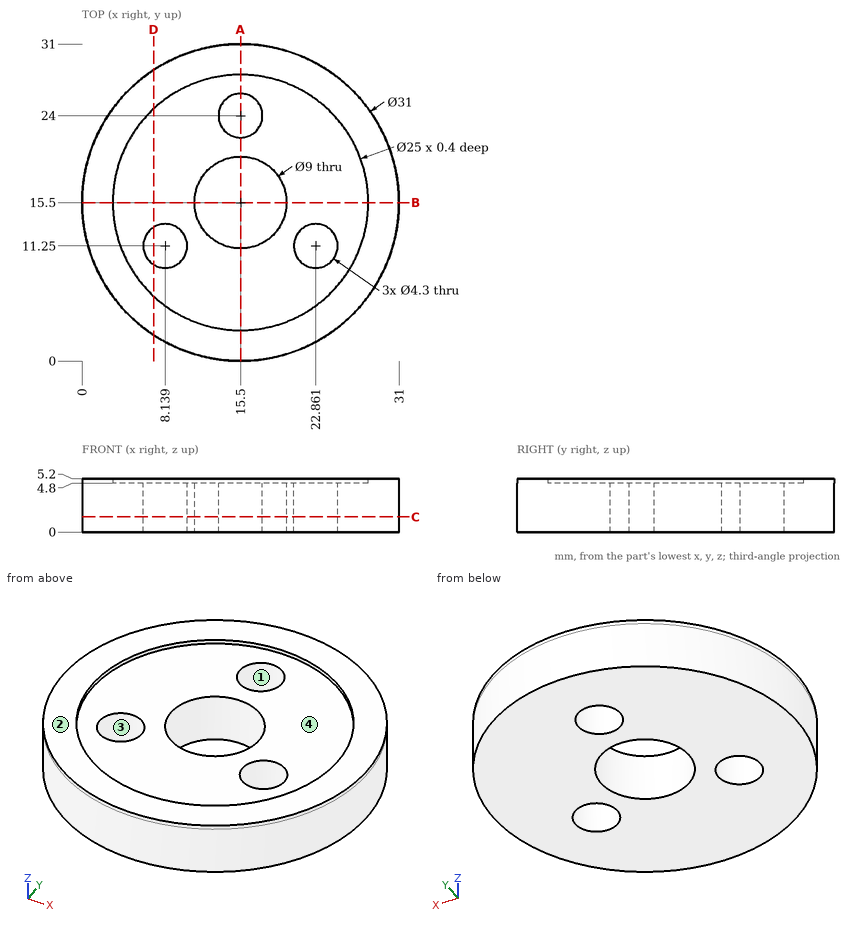
Here's the drawing with two shaded views (mm, measured from the low corner). I have some questions. A direction names the side the tool comes from. Give positions to 0.01 mm unless a question says otherwise; leave off trailing zeros. Order: outer loops, then holes, each group sorted by start corner. A loop starts at its lowest first (then second) coordinate and runs counter-clockwise, first axis right, second up. Notation, with made-up numbers: M -25,5.5 L 1,5.5 A36 ccw 1,41.5 Z; hole C -34,36 d5. An arc over 180 degrees is marked long. Answer as a JSON object with one key per item and string values. Group by question number.
1) On a 3-axis mill with a long thin cutter (end or side, diameter ignored), from which of +Z, -Z, +X, -X, +Y, -Y can I reach the whole of each face in a straight line? I mean the marked faces 3 and 4. Say none if no direction works.
2) Suppose I cut it at B-B, the plane y = 15.5. Write out the boundary of the cut face in (x, z), plus the area to 3 significant figures.
3) Suppose I cut it at D-D, the plane x = 7. Write out the boundary of the cut face in (y, z) (1 decimal), plus the area to 3 significant figures.
4) Suppose I cut it at C-C, the plane z = 1.5. Write out the boundary of the cut face in (x, y), plus the area to 3 significant figures.
5) Please list where these lines run through material, in increasing order: L1, parallel to Y at x = 15.5, z = 3.35; L2, parallel to Z at x = 25, y = 8.5; L3, parallel to X at y = 17, z = 4.5. Write a range as [from, to].
6) I'm going to push flat-ended pins straight in: pin 1 Ø2 at (x, y) = (23, 13) entering from +Z; pin 2 Ø1.5 at (x, z) = (14.5, 3.5) entering from -Y; pin 3 Ø3 at (x, z) = (8, 1.5) entering from -Y. Where does each tip first touch, or does it pass through?
7) We'd pull the mould along Y, two halves only. Please class the marked faces 1 and 2: pulls with the +Y half, pulls with the -Y half, needs draft (parallel to the pull), parting line crosses it, or undercut.
8) Suppose I cut it at A-A, the plane x = 15.5. Write out the boundary of the cut face in (y, z).
Results found:
{
 "1": {"face 3": "+Z, -Z", "face 4": "+Z"},
 "2": {"outline": "M 0,0 L 11,0 L 11,4.8 L 3,4.8 L 3,5.2 L 0,5.2 Z; M 20,0 L 31,0 L 31,5.2 L 28,5.2 L 28,4.8 L 20,4.8 Z", "area": "108 mm²"},
 "3": {"outline": "M 2.5,0 L 9.4,0 L 9.4,4.8 L 6.3,4.8 L 6.3,5.2 L 2.5,5.2 Z; M 13.1,0 L 28.5,0 L 28.5,5.2 L 24.7,5.2 L 24.7,4.8 L 13.1,4.8 Z", "area": "110 mm²"},
 "4": {"outline": "C 15.5,15.5 d31; hole C 8.14,11.25 d4.3; hole C 15.5,15.5 d9; hole C 15.5,24 d4.3; hole C 22.86,11.25 d4.3", "area": "648 mm²"},
 "5": {"L1": "[0, 11], [20, 21.85], [26.15, 31]", "L2": "[0, 4.8]", "L3": "[0.07, 11.26], [19.74, 30.93]"},
 "6": {"pin 1": "z = 4.8", "pin 2": "y = 0", "pin 3": "y = 1.21"},
 "7": {"face 1": "undercut", "face 2": "needs draft"},
 "8": {"outline": "M 0,0 L 11,0 L 11,4.8 L 3,4.8 L 3,5.2 L 0,5.2 Z; M 20,0 L 21.85,0 L 21.85,4.8 L 20,4.8 Z; M 26.15,0 L 31,0 L 31,5.2 L 28,5.2 L 28,4.8 L 26.15,4.8 Z"}
}
